For this review, use the dimensioned drawing (mm, ordinates from the lowest corner) and the shaded views. A direction names the side the tool comes from. Give positions to 0.01 mm unless a question says otherwise; leave off trailing zeros. Write each loop counter-clockwise with the first axis right and the second up, starting at its lowest first coordinate (ties: lowest second). Pieces come first, ordered by that corner, then holes. Notation, with made-up numbers: (8, 50) -> (28, 50) arc R37 cw to (28, 87) -> close; hole circle Ø11 at (-34, 10). An arc over 180 degrees is marked (long way). Write each question's results on one line, items separated by ' | '. Start each with the question number.
(1) Mouldability with a two-part tool opening along X and no side actions: class the marked faces 1, 2 and 3 as released by +X, released by -X, zero draft, split by the parting line, or undercut.
(2) Clearance check with flat-ended pins moving along their axes: pin 1 (4 mm diameter, centred on x = 31, z = 2, fed in from +Y); pin 2 (2.5 mm diameter, centred on y = 12.5, z = 2.5, fed in from +X). State where each tip first meets the part, or that it passes through.
(3) Take a section at D-D (z = 1). State the section outline as (x, y) points (1 decimal).
(4) Take a section at C-C (y = 24.5). State the section outline as (x, z) points (1 decimal).
(5) Take a section at B-B (z = 5). State the section outline as (x, y) points (1 decimal).
(6) For the marked faces 4, 5 and 6, list the 3-axis set-ups (+Z, -Z, +X, -X, +Y, -Y) from which the entire face can be reached by the end or side of a thin tool; tool diameter is ignored.
(7) To check wall thickness, follow probe 1 along X at (y, z) = (2.45, 3.81) (1 decimal); probe 2 along X at (y, z) = (21.5, 2.75) (1 decimal); probe 3 along Y at (x, z) = (3, 6.75). State the ranges of each line that lie inside material, in increasing order.
(8) Take a section at A-A (x = 3.81). State the section outline as (y, z) points.
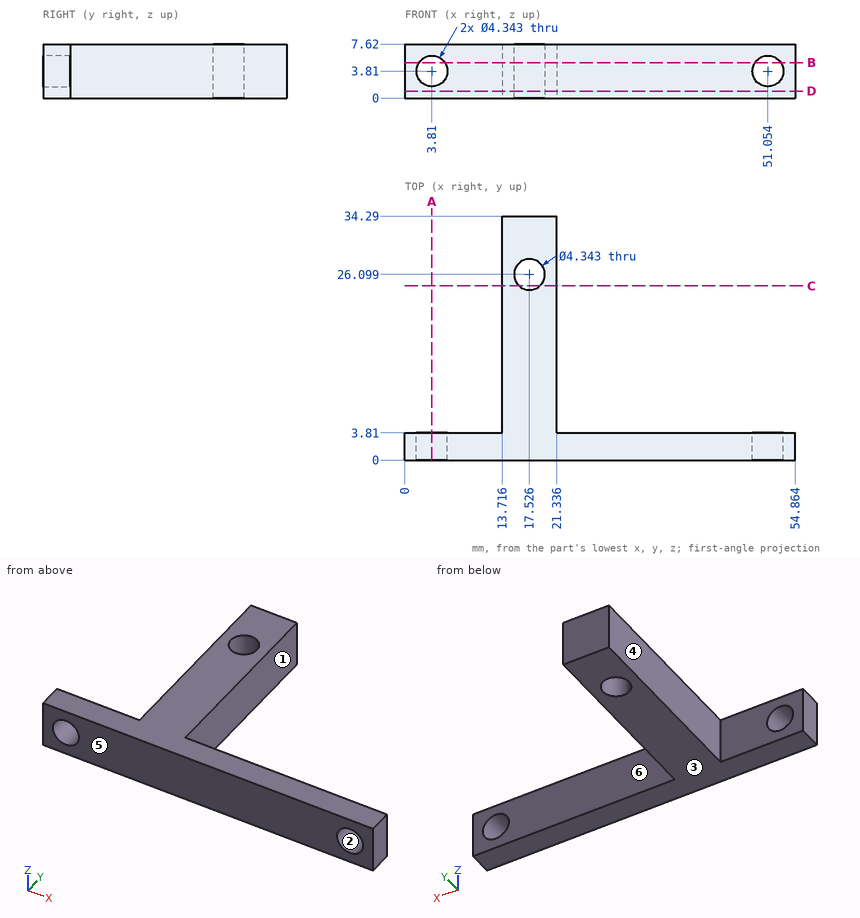
Report:
1) face 1: released by +X | face 2: undercut | face 3: zero draft
2) pin 1: y = 3.81 | pin 2: x = 21.34
3) outline: (0, 0) -> (54.9, 0) -> (54.9, 3.8) -> (21.3, 3.8) -> (21.3, 34.3) -> (13.7, 34.3) -> (13.7, 3.8) -> (0, 3.8) -> close; hole circle Ø4.3 at (17.5, 26.1)
4) outline: (13.7, 0) -> (16.1, 0) -> (16.1, 7.6) -> (13.7, 7.6) -> close; (19, 0) -> (21.3, 0) -> (21.3, 7.6) -> (19, 7.6) -> close
5) outline: (0, 0) -> (2, 0) -> (2, 3.8) -> (0, 3.8) -> close; (5.6, 0) -> (49.2, 0) -> (49.2, 3.8) -> (21.3, 3.8) -> (21.3, 34.3) -> (13.7, 34.3) -> (13.7, 3.8) -> (5.6, 3.8) -> close; (52.9, 0) -> (54.9, 0) -> (54.9, 3.8) -> (52.9, 3.8) -> close; hole circle Ø4.3 at (17.5, 26.1)
6) face 4: +Z, -Z, -X, +Y | face 5: +Z, -Z, +X, -X, -Y | face 6: +Z, -Z, +X, +Y
7) probe 1: 0 to 1.6, 6 to 48.9, 53.2 to 54.9 | probe 2: 13.7 to 21.3 | probe 3: 0 to 3.81
8) outline: (0, 0) -> (3.81, 0) -> (3.81, 1.64) -> (0, 1.64) -> close; (0, 5.98) -> (3.81, 5.98) -> (3.81, 7.62) -> (0, 7.62) -> close
